Part model, mm, in its own coordinate system. Face numbers are marked on the shaded views. A direction names the side the tool comes from. Round coordinates to 2 decimals unless told otherwise and drop trailing zeros. Loops run counter-clockwise (first coordinate to the right, second up) from the corner with the lowest first, then second, coordinate; pieces in that order, holes last. Notation, with made-up numbers: (81.5, 73) -> (99.5, 73) arc R29 ccw to (99.5, 101) -> close; hole circle Ø11 at (82, 85). An arc over 180 degrees is marked (long way). Answer as a JSON object with one key per item and string values. Group by question number.
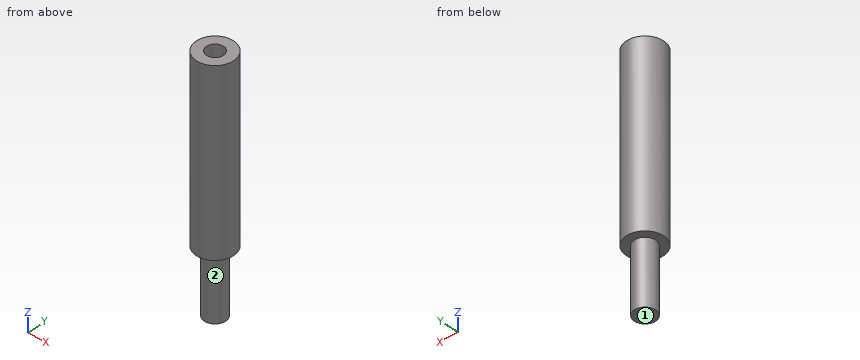
from build123d import *

# Parameters (mm, degrees)
SKETCH1_R                   = 3.5
BOSS_EXTRUDE1_DEPTH         = 33.5
SKETCH2_R                   = 2
BOSS_EXTRUDE2_DEPTH         = 12
TAP_DRILL_FOR_M3_TAP1_D     = 3.2
TAP_DRILL_FOR_M3_TAP1_DEPTH = 14
TAP_DRILL_FOR_M3_TAP1_TIP   = 0.96137699


with BuildPart() as part:
    # Sketch1 → Boss-Extrude1 (new body)
    with BuildSketch(Plane.XY):
        Circle(SKETCH1_R)
    extrude(amount=BOSS_EXTRUDE1_DEPTH)

    # Sketch2 → Boss-Extrude2 (add)
    with BuildSketch(Plane(origin=(0, 0, 0), x_dir=(-1, 0, 0), z_dir=(0, 0, -1))):
        Circle(SKETCH2_R)
    extrude(amount=BOSS_EXTRUDE2_DEPTH)

    # Tap Drill for M3 Tap1
    with Locations(Plane.XY.offset(33.5)):
        with Locations((0, 0)):
            Hole(TAP_DRILL_FOR_M3_TAP1_D / 2, depth=TAP_DRILL_FOR_M3_TAP1_DEPTH)
            with Locations((0, 0, -(TAP_DRILL_FOR_M3_TAP1_DEPTH + TAP_DRILL_FOR_M3_TAP1_TIP / 2))):  # 118° drill point
                Cone(0, TAP_DRILL_FOR_M3_TAP1_D / 2, TAP_DRILL_FOR_M3_TAP1_TIP, mode=Mode.SUBTRACT)


solid = part.part
Item 1: Which spindle directions (+Z, -Z, +X, -X, +Y, -Y) get a long thin tool onto all of the face, cutting with end or side? Do the marked faces 1 and 2. Say none if no direction does.
Item 2: Band-saw the part on A-A, the plane z = 27.5. List the corners of the cut face in (x, y), plus the area to 3 significant figures.
Item 3: Drill centre lines: line 1 (Y direction, x = 0, z = 22.5); line 2 (Z direction, x = 1.5, y = 2.75); line 3 (X direction, y = 1, z = 4). Where is each one in solid material? Low to high.
Item 4: Band-saw the part on B-B, the plane z = -4. List the corners of the cut face in (x, y).
Item 5: Drop a flat-ended pin along its axis: pin 1 Ø1.5 at (y, z) = (-2.5, 11) entering from +X. Give the stop position or say it passes through.
Item 6: Band-saw the part on D-D, the plane y = -3. List the corners of the cut face in (x, z).
Item 7: Band-saw the part on C-C, the plane x = 2.75. List the corners of the cut face in (y, z), plus the area to 3 significant figures.
Entries:
{
 "1": {"face 1": "-Z, +X, -X, +Y, -Y", "face 2": "-Z"},
 "2": {"outline": "circle Ø7 at (0, 0); hole circle Ø3.2 at (0, 0)", "area": "30.4 mm²"},
 "3": {"line 1": "-3.5 to -1.6, 1.6 to 3.5", "line 2": "0 to 33.5", "line 3": "-3.35 to 3.35"},
 "4": {"outline": "circle Ø4 at (0, 0)"},
 "5": {"pin 1": "x = 3.03"},
 "6": {"outline": "(-1.8, 0) -> (1.8, 0) -> (1.8, 33.5) -> (-1.8, 33.5) -> close"},
 "7": {"outline": "(-2.17, 0) -> (2.17, 0) -> (2.17, 33.5) -> (-2.17, 33.5) -> close", "area": "145 mm²"}
}
